```python
from build123d import *

# Parameters (mm, degrees)
F0_W     = 914.4
F0_H     = 1219.2
F1_DEPTH = 304.8
F2_T     = -19.05
F3_W     = 152.4
F3_H     = 50.8
F4_DEPTH = 1280.16
F5_R     = 5.08
F6_R     = 12.7
F7_DEPTH = 25.4


with BuildPart() as f1:
    # F0 (on Top) → F1 (new body)
    with BuildSketch(Plane.XY):
        with Locations((-5.7078478858, -19.3861435029)):
            Rectangle(F0_W, F0_H)
    extrude(amount=F1_DEPTH)

    # F2
    f2_openings = [f1.faces().sort_by_distance(p)[0] for p in [
        (-5.707848, -19.386144, 304.8),
    ]]
    offset(amount=F2_T, openings=f2_openings)

    # F3 (on face) → F4 (cut)
    with BuildSketch(Plane.XZ.offset(628.9861435029)):
        with Locations((-5.7078478858, 228.6)):
            Rectangle(F3_W, F3_H)
    extrude(amount=-F4_DEPTH, mode=Mode.SUBTRACT)

    # F5
    f5_edges = [f1.edges().sort_by_distance(p)[0] for p in [
        (-5.707848, -609.936144, 254),
        (-5.707848, -628.986144, 254),
        (-5.707848, 571.163856, 254),
        (-5.707848, 590.213856, 254),
    ]]
    fillet(f5_edges, radius=F5_R)

    # F6 (on face) → F7 (cut)
    with BuildSketch(Plane.XY.offset(19.05)):
        Circle(F6_R)
    extrude(amount=-F7_DEPTH, mode=Mode.SUBTRACT)


solid = f1.part
```
Part model, mm, in its own coordinate system. A direction names the side the tool comes from. Round coordinates to 2 decimals unless told otherwise and drop trailing zeros. Write each loop counter-clockwise with the first axis right and the second up, starting at its lowest first coordinate (ties: lowest second). Pieces come first, ordered by that corner, then holes. Notation, with made-up numbers: (24, 34.25) -> (42, 34.25) arc R14 cw to (42, 39.25) -> close; hole circle Ø11 at (19, 48.5). An arc over 180 degrees is marked (long way). Return JSON: item names as keys, results as strings. Group by question number.
Q1. Saw through at D-D on x = -139.5. Write the cut outline in (y, z), plus the area to 3 significant figures.
Q2. Pin check, flat tip, straight feed: pin 1 (12 mm diameter, centred on x = -273.5, y = 136.5, fed in from +Z). Stop position of the tip, or through.
Q3. Saw through at A-A on x = 0. Write the cut outline in (y, z).
Q4. Mould opens along Y. For faces 3 (the flat face through (-12, 590.214, 150)), 4 (the flat face through (451.492, -28, 150)), 5 (the flat face through (-12, 571.164, 160)) say: pulls with the +Y half, pulls with the -Y half, needs draft (parallel to the pull), parting line crosses it, or undercut.
Q5. Saw through at C-C on z = 141.5. Write the cut outline in (x, y), plus the area to 3 significant figures.
Q6. Which spindle directions (+Z, -Z, +X, -X, +Y, -Y) get a long thin tool onto all of the face, cutting with end or side? Do faces 1 (the flat face through (-462.908, -28, 150)), 2 (the flat face through (432.442, -28, 160)). Say none if no direction does.
Q7. Probe L1, parallel to Y at x = 94.5, z = 194; L2, parallel to X at y = 128.5, z = 267; L3, parallel to Y at x = 0, z = 8. List the from-to ranges inside material, lowest first. Write a range as [from, to].
Q8. Saw through at B-B on y = 0. Write the cut outline in (x, z), plus the area to 3 significant figures.
Answer:
{
 "1": {"outline": "(-628.99, 0) -> (590.21, 0) -> (590.21, 304.8) -> (571.16, 304.8) -> (571.16, 19.05) -> (-609.94, 19.05) -> (-609.94, 304.8) -> (-628.99, 304.8) -> close", "area": "34,100 mm2"},
 "2": {"pin 1": "z = 19.05"},
 "3": {"outline": "(-628.99, 0) -> (-12.7, 0) -> (-12.7, 19.05) -> (-609.94, 19.05) -> (-609.94, 203.2) -> (-628.99, 203.2) -> close; (-628.99, 259.08) arc R5.08 ccw to (-623.91, 254) -> (-615.02, 254) arc R5.08 ccw to (-609.94, 259.08) -> (-609.94, 304.8) -> (-628.99, 304.8) -> close; (12.7, 0) -> (590.21, 0) -> (590.21, 203.2) -> (571.16, 203.2) -> (571.16, 19.05) -> (12.7, 19.05) -> close; (571.16, 259.08) arc R5.08 ccw to (576.24, 254) -> (585.13, 254) arc R5.08 ccw to (590.21, 259.08) -> (590.21, 304.8) -> (571.16, 304.8) -> close"},
 "4": {"face 3": "pulls with the +Y half", "face 4": "needs draft", "face 5": "undercut"},
 "5": {"outline": "(-462.91, -628.99) -> (451.49, -628.99) -> (451.49, 590.21) -> (-462.91, 590.21) -> close; hole (-443.86, -609.94) -> (432.44, -609.94) -> (432.44, 571.16) -> (-443.86, 571.16) -> close", "area": "79,800 mm2"},
 "6": {"face 1": "+Z, -Z, -X, +Y, -Y", "face 2": "+Z"},
 "7": {"L1": "[-628.99, -609.94], [571.16, 590.21]", "L2": "[-462.91, -443.86], [432.44, 451.49]", "L3": "[-628.99, -12.7], [12.7, 590.21]"},
 "8": {"outline": "(-462.91, 0) -> (-12.7, 0) -> (-12.7, 19.05) -> (-443.86, 19.05) -> (-443.86, 304.8) -> (-462.91, 304.8) -> close; (12.7, 0) -> (451.49, 0) -> (451.49, 304.8) -> (432.44, 304.8) -> (432.44, 19.05) -> (12.7, 19.05) -> close", "area": "27,800 mm2"}
}
